For this review, take the finished solid that the model builds, in its own axes (mm). Round coordinates to 2 decimals unless told otherwise and drop trailing zeros. Order: outer loops, then holes, each group sorted by start corner. A loop starts at its lowest first (then second) coordinate and runs counter-clockwise, first axis right, second up. Notation, with made-up numbers: M 86.5,-25 L 102.5,-25 A7 cw 102.5,-16 Z; hole C 22,64 d10. An arc over 180 degrees is marked long. Write item = value, one per line. Start each with the question number.
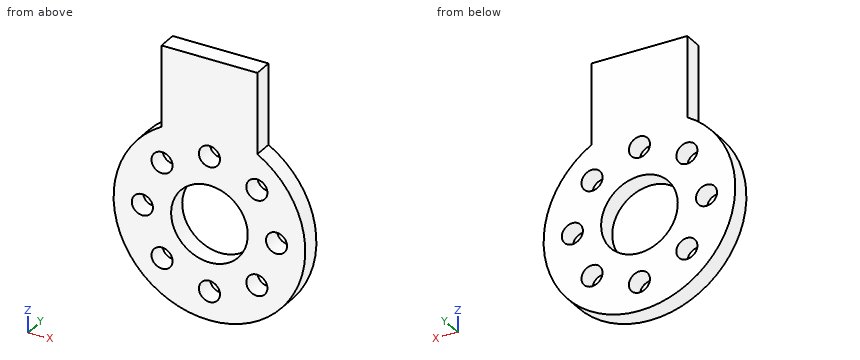
from build123d import *

# Parameters (mm, degrees)
BOSS_EXTRUDE1_DEPTH  = 5
M5_CLEARANCE_HOLE1_D = 5.5
SKETCH6_R            = 10
CUT_EXTRUDE1_DEPTH   = 50.773304207


with BuildPart() as part:
    # Sketch1 → Boss-Extrude1 (new body)
    with BuildSketch(Plane(origin=(0, 0, 0), x_dir=(1, 0, 0), z_dir=(0, 1, 0))):
        with BuildLine():
            Line((-12.5, -42.747886634), (12.5, -42.747886634))
            Line((12.5, -42.747886634), (12.5, -21.650635095))
            ThreePointArc((12.5, -21.650635095), (0, 25), (-12.5, -21.650635095))
            Line((-12.5, -21.650635095), (-12.5, -42.747886634))
        make_face()
    extrude(amount=BOSS_EXTRUDE1_DEPTH)

    # M5 Clearance Hole1 (through all)
    with Locations(Plane(origin=(0, 5, 0), x_dir=(1, 0, 0), z_dir=(0, 1, 0))):
        with Locations((-12.374368671, 12.374368671), (0, 17.5), (12.374368671, 12.374368671), (17.5, 0), (12.374368671, -12.374368671), (0, -17.5), (-12.374368671, -12.374368671), (-17.5, 0)):
            Hole(M5_CLEARANCE_HOLE1_D / 2)

    # Sketch6 → Cut-Extrude1 (cut, through all)
    with BuildSketch(Plane(origin=(0, 5, 0), x_dir=(1, 0, 0), z_dir=(0, 1, 0))):
        with Locations(Location((0, 0, 0), (0, 0, 270))):
            Circle(SKETCH6_R)
    extrude(amount=-CUT_EXTRUDE1_DEPTH, mode=Mode.SUBTRACT)


solid = part.part
(1) We need section D-D, the plane x = -6.5. Write out the cut boundary in (y, z).
(2) For line 1 along Z through (x, y) = (13.5, 2); line 2 along X through (y, z) = (2.5, 18); line 3 along Z through (x, y) = (20, 1.15), list the stretches that pass through material, from the lowest coordinate up.
(3) We need section A-A, the plane z = 0. Write out the cut boundary in (x, y).
(4) We need section C-C, the plane z = 7.5. Write out the cut boundary in (x, y), then the cut area to 3 significant figures.
(5) Insertion check: pin 1 (1.5 mm diameter, centred on x = -14, y = 3.5, fed in from +Z); pin 2 (1.5 mm diameter, centred on y = 3.5, z = 31, fed in from +X); pin 3 (3 mm diameter, centred on x = -2, y = 1, fed in from -Z) (3 decimals). Each pin has a flat end and moves straight along its axis. Give the tip position at first contact, or say it passes through.
(6) We need section B-B, the plane x = 0. Write out the cut boundary in (y, z).
Values:
q1.outline = M 0,-24.14 L 5,-24.14 L 5,-7.6 L 0,-7.6 Z; M 0,7.6 L 5,7.6 L 5,42.75 L 0,42.75 Z
q2.line_1 = -21.04 to -14.88, -9.87 to 9.87, 14.88 to 21.04
q2.line_2 = -17.35 to -2.7, 2.7 to 17.35
q2.line_3 = -15 to -1.15, 1.15 to 15
q3.outline = M -25,0 L -20.25,0 L -20.25,5 L -25,5 Z; M -14.75,0 L -10,0 L -10,5 L -14.75,5 Z; M 10,0 L 14.75,0 L 14.75,5 L 10,5 Z; M 20.25,0 L 25,0 L 25,5 L 20.25,5 Z
q4.outline = M -23.85,0 L -6.61,0 L -6.61,5 L -23.85,5 Z; M 6.61,0 L 23.85,0 L 23.85,5 L 6.61,5 Z
q4.area = 172 mm²
q5.pin_1 = 21.2
q5.pin_2 = 12.5
q5.pin_3 = -24.995
q6.outline = M 0,-25 L 5,-25 L 5,-20.25 L 0,-20.25 Z; M 0,-14.75 L 5,-14.75 L 5,-10 L 0,-10 Z; M 0,10 L 5,10 L 5,14.75 L 0,14.75 Z; M 0,20.25 L 5,20.25 L 5,42.75 L 0,42.75 Z
